```python
from build123d import *

# Parameters (mm, degrees)
ESQUISSE2_W             = 1.3
ESQUISSE2_H             = 0.5
CONG_1_R                = 1
CHANFREIN1_SIZE         = 1
ESQUISSE3_R             = 3.7
ENL_V_MAT_EXTRU_1_DEPTH = 10
ESQUISSE4_R             = 3
ESQUISSE4_R_2           = 2.5
ENL_V_MAT_EXTRU_2_DEPTH = 196.961730958
ESQUISSE6_W             = 1.3
ESQUISSE6_H             = 0.5


with BuildPart() as part:
    # Esquisse1 → Base-Révolution (revolve)
    with BuildSketch(Plane.XY, mode=Mode.PRIVATE) as base_r_volution_sk:
        Polygon((0, 0), (0, 24), (18, 24), (18, 12), (50, 12), (50, 10), (62, 10), (62, 9), (128, 9), (128, 10), (143, 10), (143, 9), (193, 9), (193, 0), align=None)
    revolve(base_r_volution_sk.sketch.rotate(Axis((-48.771720193, 0, 0), (1, 0, 0)), 90), axis=Axis((-48.771720193, 0, 0), (1, 0, 0)))

    # Esquisse2 → Enlèvement de matière-Révolution1 (revolve, cut)
    with BuildSketch(Plane.XY, mode=Mode.PRIVATE) as enl_vement_de_mati_re_r_volution1_sk:
        with Locations((47.65, 11.75)):
            Rectangle(ESQUISSE2_W, ESQUISSE2_H)
    revolve(enl_vement_de_mati_re_r_volution1_sk.sketch.rotate(Axis((0, 0, 0), (1, 0, 0)), 90), axis=Axis((0, 0, 0), (1, 0, 0)), mode=Mode.SUBTRACT)

    # Congé1
    cong_1_edges = [part.edges().sort_by_distance(p)[0] for p in [
        (62, 0, -9),
        (128, 0, -9),
    ]]
    fillet(cong_1_edges, radius=CONG_1_R - 0.0001)  # a hair under: the kernel refuses the full size

    # Chanfrein1
    chanfrein1_edges = [part.edges().sort_by_distance(p)[0] for p in [
        (193, 0, -9),
        (18, 0, -24),
        (0, 0, -24),
    ]]
    chamfer(chanfrein1_edges, length=CHANFREIN1_SIZE)

    # Esquisse3 → Enlèv. mat.-Extru.1 (cut, symmetric)
    with BuildSketch(Plane.XY):
        with Locations((161, 0)):
            Circle(ESQUISSE3_R)
    extrude(amount=ENL_V_MAT_EXTRU_1_DEPTH, both=True, mode=Mode.SUBTRACT)

    # Esquisse4 → Enlèv. mat.-Extru.2 (cut, through all)
    with BuildSketch(Plane.ZY):
        with Locations((7, 16)):
            Circle(ESQUISSE4_R)
        with Locations((7, -16)):
            Circle(ESQUISSE4_R)
        with Locations((16, 0)):
            Circle(ESQUISSE4_R_2)
    extrude(amount=-ENL_V_MAT_EXTRU_2_DEPTH, mode=Mode.SUBTRACT)

    # Esquisse6 → Enlèvement de matière-Révolution2 (revolve, cut)
    with BuildSketch(Plane.XY, mode=Mode.PRIVATE) as enl_vement_de_mati_re_r_volution2_sk:
        with Locations((140.65, 9.75)):
            Rectangle(ESQUISSE6_W, ESQUISSE6_H)
    revolve(enl_vement_de_mati_re_r_volution2_sk.sketch.rotate(Axis((141.562186711, 0, 0), (1, 0, 0)), 90), axis=Axis((141.562186711, 0, 0), (1, 0, 0)), mode=Mode.SUBTRACT)


solid = part.part
```
Check sheet for the modelled part. Datum: model origin and axes. Units: mm. A direction names the side the tool comes from. Coordinates: 2 decimals unless noted, no trailing zeros. Write each loop counter-clockwise with the first axis right and the second up, starting at its lowest first coordinate (ties: lowest second). Pieces come first, ordered by that corner, then holes. Notation, with made-up numbers: (88, 37.5) - (104, 37.5) arc R31 cw to (104, 67.5) - close; hole circle Ø3 at (15.5, 61). An arc over 180 degrees is marked (long way). One line per question, with ' | ' between items.
Item 1: Sectioned sample at A-A on x = 161. Record the boundary of the cut face in (y, z), plus the area to 3 significant figures.
Determined:
outline: (-3.7, -8.2) - (-3.7, 8.2) arc R9 ccw to start; (3.7, -8.2) arc R9 ccw to (3.7, 8.2) - close | area: 125 mm2
Item 2: Gauge pin test, flat ends, axial feed: P1, Ø5, axis at x = 127, y = 1, coming from the +Z side; P2, Ø12, axis at x = 161, y = 0, coming from the -Z side; P3, Ø10, axis at x = 20.5, z = -12, coming from the +Y side. Record the tip position at first contact, or that the pin passes through.
Determined:
P1: stops at z = 10 | P2: stops at z = -9 | P3: stops at y = 22.47
Item 3: Thickness scan on line 1 (Y direction, x = 13, z = 7); line 2 (X direction, y = -13, z = 6.5); line 3 (Y direction, x = 161, z = -0.75). Record the ranges inside material, lowest first. Write a range as [from, to].
Determined:
line 1: y = [-22.96, -19], [-13, 13], [19, 22.96] | line 2: x = [0, 18] | line 3: y = [-8.97, -3.7], [3.7, 8.97]
Item 4: Access from +Z, -Z, +X, -X, +Y, -Y to the whole of each face (thin tool, end or side, straight path). Record for faces 1 (the face through (140.659, 9.274, -2.059)), 2 (the face through (142, 0, -10)), 3 (the face through (8.874, 13.338, 8.384)).
Determined:
face 1: none | face 2: +X | face 3: +X, -X
Item 5: Mould release check, pull along Z, two halves, no side actions. Record for faces 4 (the face through (48.3, 10, -6)), 5 (the face through (8.9, 0.1, 13.5)), 6 (the face through (56, 0, -10)): pulls with the +Z half, pulls with the -Z half, needs draft (parallel to the pull), parting line crosses it, or undercut.
Determined:
face 4: needs draft | face 5: undercut | face 6: parting line crosses it
